The model under review builds one solid part; all positions refer to its coordinate system, in mm. Face numbers are marked on the shaded views. A direction names the side the tool comes from. Coordinates: 2 decimals unless noted, no trailing zeros. Loops run counter-clockwise (first coordinate to the right, second up) from the corner with the lowest first, then second, coordinate; pieces in that order, holes last. Notation, with made-up numbers: M 4,73.25 L 17,73.25 A28 cw 17,104.25 Z; hole C 88,-28 d9. An arc over 180 degrees is marked long. One line per item, written item: value.
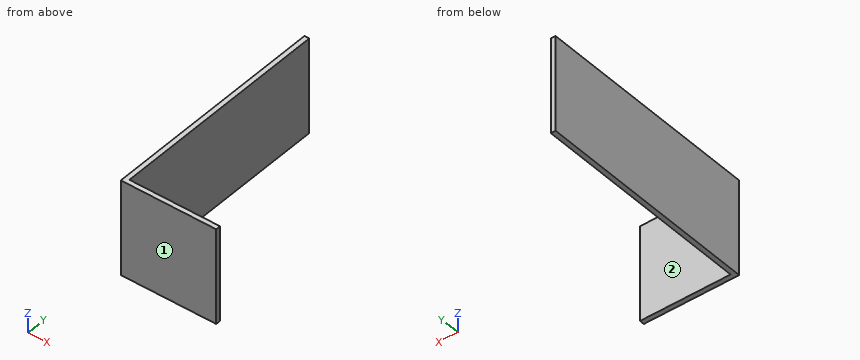
```python
from build123d import *

# Parameters (mm, degrees)
F0_W     = 500
F0_H     = 50
F0_H_2   = 224.9779105186
F0_H_3   = 225.0220894814
F1_DEPTH = 30
F2_W     = 30
F2_H     = 600
F3_DEPTH = 1400


with BuildPart() as f1:
    # F0 (on Front) → F1 (new body)
    with BuildSketch(Plane.XZ):
        Polygon((0, 600), (0, 0), (50, 0), (50, 50), (50, 275.0220894814), (50, 325.0220894814), (50, 550), (50, 600), align=None)
        with Locations((300, 575)):
            Rectangle(F0_W, F0_H)
        with Locations((300, 437.5110447407)):
            Rectangle(F0_W, F0_H_2)
        with Locations((300, 300.0220894814)):
            Rectangle(F0_W, F0_H)
        with Locations((300, 162.5110447407)):
            Rectangle(F0_W, F0_H_3)
        with Locations((300, 25)):
            Rectangle(F0_W, F0_H)
        Polygon((550, 50), (550, 0), (600, 0), (600, 600), (550, 600), (550, 550), (550, 325.0220894814), (550, 275.0220894814), align=None)
    extrude(amount=-F1_DEPTH)

    # F2 (on face) → F3 (join)
    with BuildSketch(Plane(origin=(0, 30, 0), x_dir=(-1, 0, 0), z_dir=(0, 1, 0))):
        with Locations((-15, 300)):
            Rectangle(F2_W, F2_H)
    extrude(amount=F3_DEPTH)


solid = f1.part
```
(1) Insertion check: pin 1 Ø1.5 at (y, z) = (762.5, 432) entering from +X; pin 2 Ø6 at (x, z) = (527.5, 346.5) entering from +Y. Each pin has a flat end and moves straight along its axis. Give the tip position at first contact, or say it passes through.
Checks:
pin 1: x = 30
pin 2: y = 30
(2) Add section A-A on z = 349. State the section outline as (x, y) points, then the cut area to 3 significant figures.
Checks:
outline: M 0,0 L 600,0 L 600,30 L 30,30 L 30,1430 L 0,1430 Z
area: 60,000 mm^2
(3) Tool access review of the marked faces 1 and 2: name each direction out of +Z, -Z, +X, -X, +Y, -Y from which nothing blocks a thin tool from reaching the whole face with its end or side.
Checks:
face 1: +Z, -Z, +X, -X, -Y
face 2: +Z, -Z, +X, +Y
(4) Add section B-B on x = 111. State the section outline as (y, z) points, then the cut area to 3 significant figures.
Checks:
outline: M 0,0 L 30,0 L 30,600 L 0,600 Z
area: 18,000 mm^2
(5) To check wall thickness, follow L1, parallel to X at y = 542.5, z = 559.5. State the ranges of the line that lie inside material, in increasing order. Write a range as [from, to].
Checks:
L1: [0, 30]
